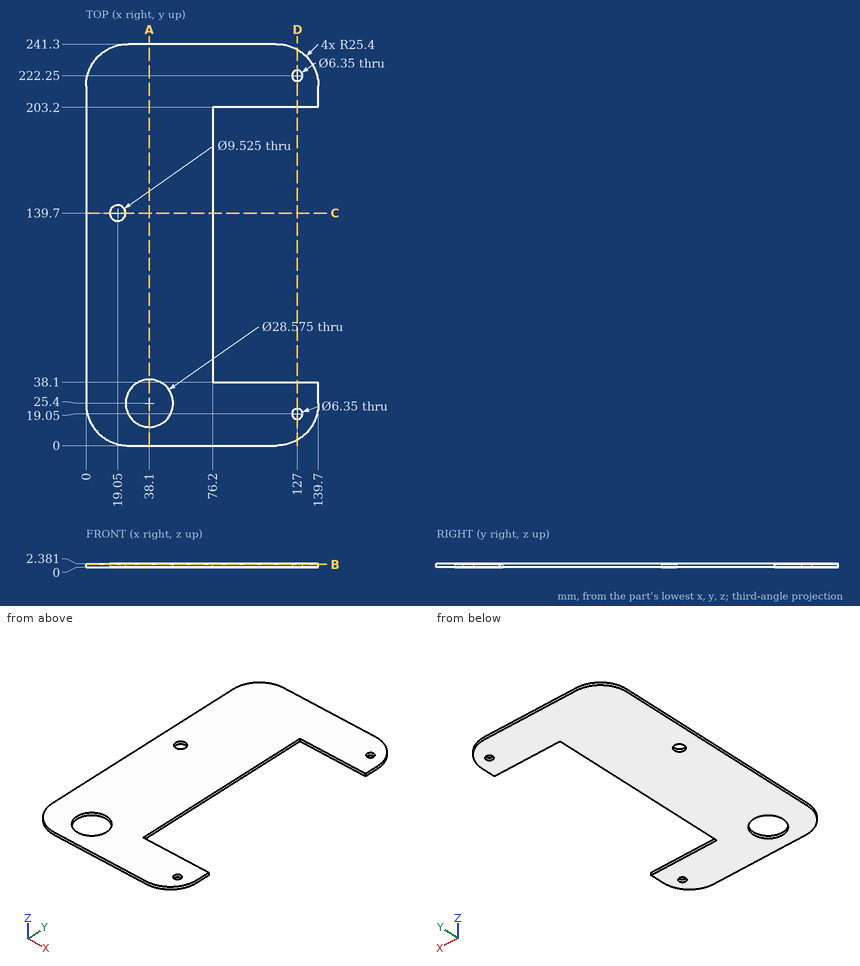
Job drawing, mm, ordinate dimensions from the low corner. One solid piece. Coordinates: 2 decimals unless noted, no trailing zeros. Write each loop counter-clockwise with the first axis right and the second up, starting at its lowest first coordinate (ties: lowest second). Pieces come first, ordered by that corner, then holes.
Item 1: Probe line 1 (Y direction, x = 126, z = 1) (1 decimal); line 2 (Y direction, x = 38.1, z = 0.65); line 3 (Y direction, x = 127, z = 1.35) (1 decimal). List the from-to ranges inside material, lowest first.
Item 2: Pin check, flat tips, straight feed: pin 1 (0.7 mm diameter, centred on y = 148.5, z = 0.5, fed in from +X); pin 2 (5.5 mm diameter, centred on x = 19.05, y = 139.7, fed in from -Z). Stop position of each tip, or through.
Item 3: Slice it at D-D (x = 127). Write the cut outline in (y, z) (1 decimal).
Item 4: Slice it at C-C (y = 139.7). Write the cut outline in (x, z), and give its area (3 significant figures).
Item 5: Slice it at A-A (x = 38.1). Write the cut outline in (y, z).
Item 6: Slice it at B-B (z = 1.9). Count the separate pieces of the cut face and the enclosed holes in it, and give its area (3 significant figures).
Results found:
1. line 1: y = 2.9 to 16, 22.1 to 38.1, 203.2 to 219.2, 225.3 to 238.4
1. line 2: y = 0 to 11.11, 39.69 to 241.3
1. line 3: y = 3.4 to 15.9, 22.2 to 38.1, 203.2 to 219.1, 225.4 to 237.9
2. pin 1: stops at x = 76.2
2. pin 2: passes through
3. outline: (3.4, 0) - (15.9, 0) - (15.9, 2.4) - (3.4, 2.4) - close; (22.2, 0) - (38.1, 0) - (38.1, 2.4) - (22.2, 2.4) - close; (203.2, 0) - (219.1, 0) - (219.1, 2.4) - (203.2, 2.4) - close; (225.4, 0) - (237.9, 0) - (237.9, 2.4) - (225.4, 2.4) - close
4. outline: (0, 0) - (14.29, 0) - (14.29, 2.38) - (0, 2.38) - close; (23.81, 0) - (76.2, 0) - (76.2, 2.38) - (23.81, 2.38) - close
4. area: 159 mm2
5. outline: (0, 0) - (11.11, 0) - (11.11, 2.38) - (0, 2.38) - close; (39.69, 0) - (241.3, 0) - (241.3, 2.38) - (39.69, 2.38) - close
6. separate pieces: 1
6. enclosed holes: 4
6. area: 21,900 mm2
